Design review of the part built by this model. Coordinates are the model's own, in mm. A direction names the side the tool comes from. Round coordinates to 2 decimals unless told otherwise and drop trailing zeros. Loops run counter-clockwise (first coordinate to the right, second up) from the corner with the lowest first, then second, coordinate; pieces in that order, holes last. Notation, with made-up numbers: (-7, 41.5) - (34, 41.5) arc R11 ccw to (34, 52.5) - close; hole circle Ø6 at (9, 77). An arc over 180 degrees is marked (long way). Return JSON: item names as keys, results as strings. Group by question number.
(1) For faces 4 (the cylindrical face through (0.266, -42.755, 3.757)), 5 (the cylindrical face through (22.035, -10.465, 4.408)), 6 (the cylindrical face through (0.23, -36.62, 3.76)), list the 3-axis set-ups (+Z, -Z, +X, -X, +Y, -Y) from which the entire face can be reached by the end or side of a thin tool; tool diameter is ignored.
(2) We need section C-C, the plane z = 1.75. Give the number of separate pieces and of enclosed holes in the cut face, and give its area (3 significant figures).
(3) Clearance check with flat-ended pins moving along their axes: pin 1 (2 mm diameter, centred on x = -7.37, y = 39.05, fed in from +Z); pin 2 (1 mm diameter, centred on x = 10.5, z = 6, fed in from +Y); pin 3 (3 mm diameter, centred on x = 14.5, z = 6, fed in from -Y); pin 4 (2 mm diameter, centred on x = 5, z = 1.5, fed in from -Y). State where each tip first meets the part, or that it passes through.
(4) We need section A-A, the plane y = 25. Write out the cut boundary in (x, z) (3 decimals).
(5) We need section D-D, the plane x = 20. Write out the cut boundary in (y, z).
(6) The part is to be moulded in two halves that separate along Y. For faces 1 (the flat face through (-20.8, 0.2, 0)), 2 (the cylindrical face through (-0.489, 42.818, 3.757)), 3 (the cylindrical face through (-7.519, 37.927, 3.757)), say which applies: pulls with the +Y half, pulls with the -Y half, needs draft (parallel to the pull), parting line crosses it, or undercut.
(7) Wall thickness on L1, parallel to X at y = -31, z = 6.5 (3 decimals); L2, parallel to X at y = -32, z = 6.25; L3, parallel to Y at x = -22, z = 0.5: over which ranges is each line inside the solid? List them lowest first. Write a range as [from, to].
(8) We need section B-B, the plane y = 0. Write out the cut boundary in (x, z) (3 decimals).
Autodesk Inventor part; units mm, degrees
ref_plane "YZ Plane" through (0, 0, 0) normal (1, 0, 0) x (0, 1, 0)
ref_plane "XZ Plane" through (0, 0, 0) normal (0, 1, 0) x (-1, 0, 0)
ref_plane "XY Plane" through (0, 0, 0) normal (0, 0, 1) x (1, 0, 0)
sketch "Sketch1" plane through (0, 0, 0) normal (0, 0, 1) x (1, 0, 0)
  arc A0 (25.273, 34.559) -> (0.0081, 42.8141) centre (0, 0) ccw
  line L0 (25.273, 34.559) -> (25.273, 0)
  line L1 (18.923, 0) -> (18.923, 31.5055)
  arc A1 (18.923, 31.5055) -> (0.0081, 36.4641) centre (-0.083, -2.439) ccw
  arc A2 (23.2283, 0) -> (20.9677, 0) centre (22.098, 0) ccw
  circle A3 centre (22.098, 32.4528) radius 1.1303
  circle A4 centre (22.098, 16.1968) radius 1.1303
  circle A5 centre (7.372, 39.0479) radius 1.1303
  arc A6 (-20.9677, 0) -> (-23.2283, 0) centre (-22.098, 0) ccw
  circle A7 centre (-22.098, 16.1968) radius 1.1303
  circle A8 centre (-22.098, 32.4528) radius 1.1303
  circle A9 centre (-7.372, 39.0479) radius 1.1303
  arc A10 (-0.0081, 36.4641) -> (-18.923, 31.5055) centre (0.083, -2.439) ccw
  arc A11 (-0.0081, 42.8141) -> (-25.273, 34.559) centre (0, 0) ccw
  line L2 (-25.273, 34.559) -> (-25.273, 0)
  line L3 (-18.923, 0) -> (-18.923, 31.5055)
  line L4 (25.273, -34.559) -> (25.273, 0)
  arc A12 (0.0081, -42.8141) -> (25.273, -34.559) centre (0, 0) ccw
  arc A13 (-25.273, -34.559) -> (-0.0081, -42.8141) centre (0, 0) ccw
  line L5 (-25.273, -34.559) -> (-25.273, 0)
  line L6 (-18.923, 0) -> (-18.923, -31.5055)
  arc A14 (-18.923, -31.5055) -> (-0.0081, -36.4641) centre (0.083, 2.439) ccw
  arc A15 (0.0081, -36.4641) -> (18.923, -31.5055) centre (-0.083, 2.439) ccw
  line L7 (18.923, 0) -> (18.923, -31.5055)
  arc A16 (-23.2283, 0) -> (-20.9677, 0) centre (-22.098, 0) ccw
  circle A17 centre (-22.098, -16.1968) radius 1.1303
  circle A18 centre (-22.098, -32.4528) radius 1.1303
  circle A19 centre (-7.372, -39.0479) radius 1.1303
  circle A20 centre (7.372, -39.0479) radius 1.1303
  circle A21 centre (22.098, -32.4528) radius 1.1303
  circle A22 centre (22.098, -16.1968) radius 1.1303
  arc A23 (20.9677, 0) -> (23.2283, 0) centre (22.098, 0) ccw
  point P0 (0, 29.76)
  point P1 (9.9838, 29.1027)
  point P2 (9.9839, 22.365)
  point P3 (9.9841, 15.6273)
  point P4 (9.9842, 8.8896)
  point P5 (9.9844, 2.1519)
  point P6 (-17.2373, 0)
  point P7 (-17.2389, 0)
  point P8 (-17.2362, -2.4348)
  point P9 (9.9845, -4.5858)
  point P10 (9.9847, -11.3235)
  point P11 (9.9848, -18.0612)
  point P12 (9.9849, -24.7989)
  point P13 (-0.4822, -30.8495)
  point P14 (0, -28.8424)
  point P15 (-10.2647, -28.1682)
  point P16 (-10.2649, -21.4305)
  point P17 (-10.265, -14.6929)
  point P18 (-10.2652, -7.9552)
  point P19 (-10.2653, -1.2175)
  point P20 (-10.2655, 5.5201)
  point P21 (-10.2656, 12.2578)
  point P22 (-10.2657, 18.9955)
  point P23 (-10.2659, 25.7332)
  point P24 (0.294, 31.7784)
  dimension "d1" = 6.35
  dimension "d2" = 2.2606
  dimension "d3" = 2.2606
  dimension "d4" = 2.2606
  dimension "d6" = 2.2606
sketch "Sketch4" plane through (0, 0, 0) normal (0, 0, 1) x (1, 0, 0)
  line L0 (-18.985, 31.3156) -> (-18.985, -31.5153)
  line L1 (18.8873, 31.3156) -> (18.8873, -31.5153)
  line L2 (-25.3178, 34.4199) -> (-25.3178, -34.6195)
  line L3 (25.0959, 34.4199) -> (25.0959, -34.6195)
  arc A0 (18.8873, 31.3156) -> (-18.985, 31.3156) centre (-0.0488, -1.3553) ccw
  arc A1 (-18.985, -31.5153) -> (18.8873, -31.5153) centre (-0.0488, 1.0453) ccw
  arc A2 (25.0959, 34.4199) -> (-25.3178, 34.4199) centre (-0.1109, 0.7967) ccw
  arc A3 (-25.3178, -34.6195) -> (25.0959, -34.6195) centre (-0.1109, 0.3555) ccw
  point P0 (0, 0)
extrude "Extrusion1" add sketch "Sketch4" along normal blind 7.62
extrude "Extrusion2" cut sketch "Sketch1" along normal blind 7.62
sketch "Sketch5" plane through (25.0959, -34.6195, 0) normal (1, 0, 0) x (0, 0, -1)
  line L0 (-7.62, 3.1043) -> (-7.62, 65.9351)
  line L1 (-6.35, 27.8057) -> (-6.0293, 27.8057)
  line L2 (-3.4893, 25.2657) -> (-3.4893, 26.1098)
  line L3 (-6.0293, 23.5698) -> (-6.35, 23.5698)
  line L4 (-6.35, 23.5698) -> (-6.35, 27.8057)
  arc A0 (-3.4893, 25.2657) -> (-6.0293, 27.8057) centre (-6.0293, 25.2657) ccw
  arc A1 (-6.0293, 23.5698) -> (-3.4893, 26.1098) centre (-6.0293, 26.1098) ccw
  point P0 (0, 34.6195)
  point P1 (-3.5246, 25.6877)
  dimension "d16" = 2.54
  dimension "d17" = 1.27
extrude "Extrusion3" cut sketch "Sketch5" against normal blind 12.7 contours L1 A0 A1 L3 L4
properties part number "new_retainer_full_cap"
Solutions:
{
 "1": {"face 4": "+Z, -Z, -Y", "face 5": "+X", "face 6": "+Z, -Z"},
 "2": {"separate pieces": "1", "enclosed holes": "15", "area": "1,350 mm^2"},
 "3": {"pin 1": "through", "pin 2": "y = 41.58", "pin 3": "y = -40.71", "pin 4": "y = -42.56"},
 "4": {"outline": "(-25.318, 0) - (-18.985, 0) - (-18.985, 7.62) - (-25.318, 7.62) - close; (18.887, 0) - (25.096, 0) - (25.096, 7.62) - (18.887, 7.62) - close"},
 "5": {"outline": "(-37.78, 0) - (37.69, 0) - (37.69, 7.62) - (-37.78, 7.62) - close; hole (-11.05, 6.03) arc R2.54 ccw to (-8.93, 3.52) arc R2.54 ccw to (-6.81, 6.03) - (-6.81, 6.35) - (-11.05, 6.35) - close"},
 "6": {"face 1": "needs draft", "face 2": "pulls with the +Y half", "face 3": "undercut"},
 "7": {"L1": "[-25.318, -18.985], [18.887, 25.096]", "L2": "[-25.32, -23.13], [-21.06, -18.13], [18.03, 21.06], [23.13, 25.1]", "L3": "[-36.79, -33.58], [-31.33, -17.32], [-15.07, -1.13], [1.13, 15.07], [17.32, 31.33], [33.58, 36.67]"},
 "8": {"outline": "(-25.318, 0) - (-23.228, 0) - (-23.228, 7.62) - (-25.318, 7.62) - close; (-20.968, 0) - (-18.985, 0) - (-18.985, 7.62) - (-20.968, 7.62) - close; (18.887, 0) - (20.968, 0) - (20.968, 7.62) - (18.887, 7.62) - close; (23.228, 0) - (25.096, 0) - (25.096, 7.62) - (23.228, 7.62) - close"}
}
